Can you work these out from the drawing? Everything is in mm from the part's minimum corner. Round coordinates to 2 decimals unless told otherwise and drop trailing zeros. Loops run counter-clockwise (first coordinate to the right, second up) from the corner with the lowest first, then second, coordinate; pieces in that order, holes last. Notation, with made-up numbers: (-13, 69.25) - (39, 69.25) arc R36 ccw to (39, 103.25) - close; hole circle Ø6 at (55, 20.5). An arc over 180 degrees is marked (long way). Answer as a JSON object with one key per item and string values. Group by question number.
1) If we mould it in two halves opening along Z, with no side actions, what happens to the marked faces 1, 2, 3 and 4? For each: pulls with the +Z half, pulls with the -Z half, needs draft (parallel to the pull), parting line crosses it, or undercut.
2) I want a section at B-B, the plane y = 18. Please give me the cut outline in (x, z), then the cut area to 3 significant figures.
3) I want a section at A-A, the plane y = 31. Please give me the cut outline in (x, z).
4) If I drill on line 1 along Z through (x, y) = (4.4, 15) (1 decimal); line 2 along Z through (x, y) = (2, 30); line 3 along Z through (x, y) = (2.25, 12), over which ranges is the centre line in solid material (lowest first)? Write a range as [from, to].
5) I want a section at C-C, the plane x = 4.65. Please give me the cut outline in (y, z).
6) Will these pins go through, and if not, where does the flat tip stop? P1, Ø1.5, axis at y = 27.5, z = 1.5, coming from the -X side; P2, Ø3, axis at y = 16, z = 0.5, coming from the +X side.
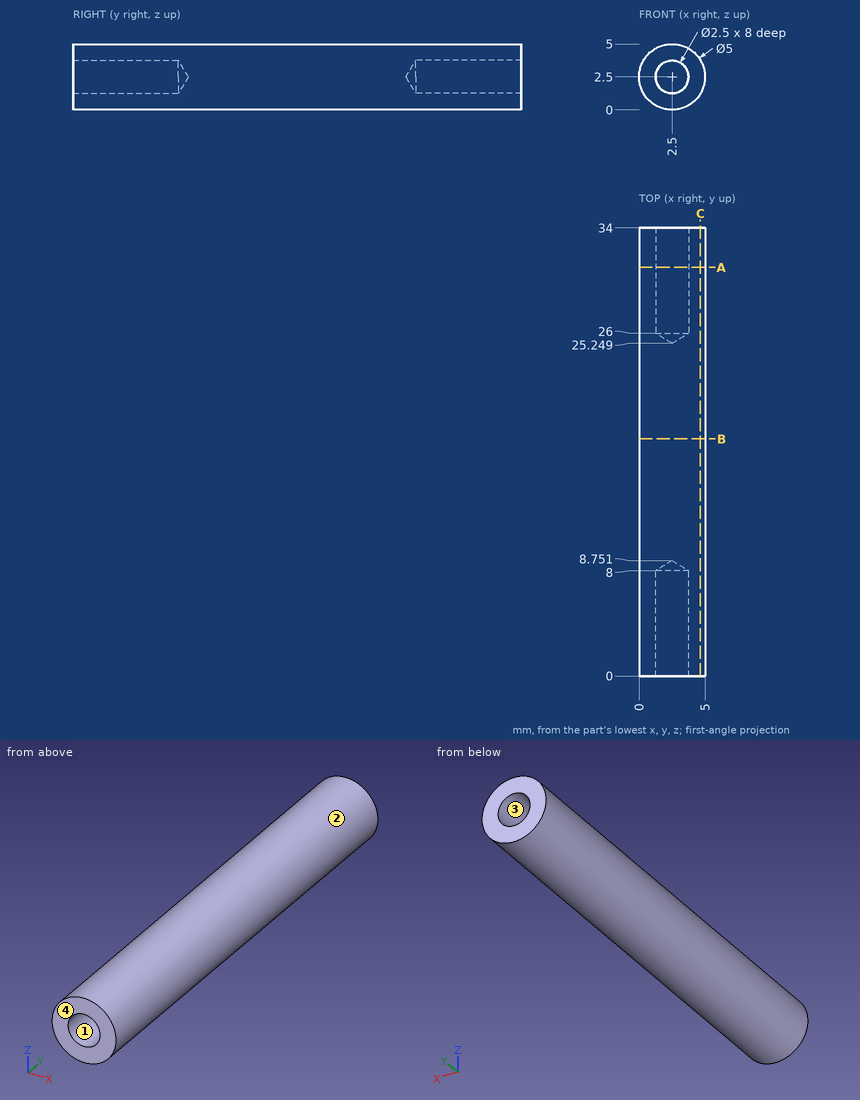
Outcome:
{
 "1": {"face 1": "undercut", "face 2": "parting line crosses it", "face 3": "undercut", "face 4": "needs draft"},
 "2": {"outline": "circle Ø5 at (2.5, 2.5)", "area": "19.6 mm^2"},
 "3": {"outline": "circle Ø5 at (2.5, 2.5); hole circle Ø2.5 at (2.5, 2.5)"},
 "4": {"line 1": "[0.9, 4.1]", "line 2": "[0.05, 1.35], [3.65, 4.95]", "line 3": "[0.01, 4.99]"},
 "5": {"outline": "(0, 1.22) - (34, 1.22) - (34, 3.78) - (0, 3.78) - close"},
 "6": {"P1": "x = 0.01", "P2": "x = 4.95"}
}
